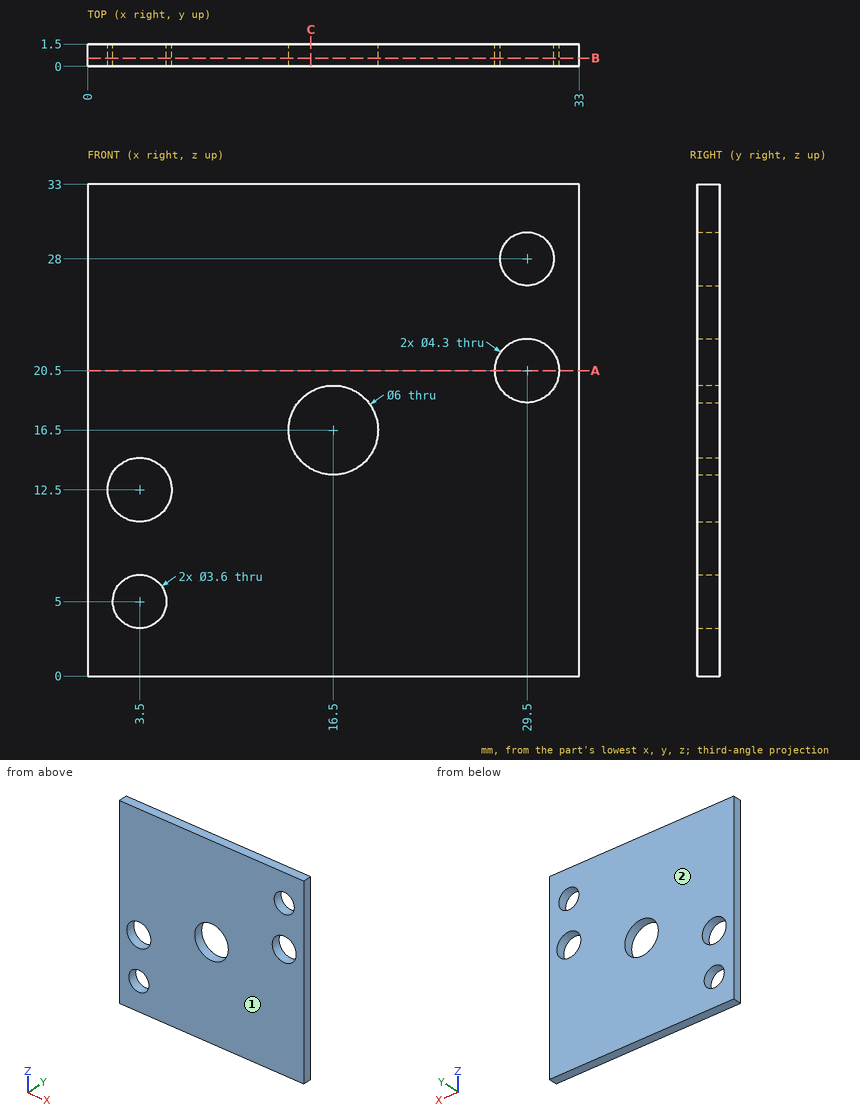
Check sheet for the drawn part. Datum: minimum x, y, z corner. Units: mm. Round coordinates to 2 decimals unless told otherwise and drop trailing zeros. Loops run counter-clockwise (first coordinate to the right, second up) from the corner with the lowest first, then second, coordinate; pieces in that order, holes last.
Item 1: Mould release check, pull along Y, two halves, no side actions. Record for the marked faces 1 and 2: pulls with the +Y half, pulls with the -Y half, needs draft (parallel to the pull), parting line crosses it, or undercut.
Item 2: Gauge pin test, flat ends, axial feed: pin 1 (4 mm diameter, centred on x = 29.5, z = 20.5, fed in from -Y); pin 2 (6 mm diameter, centred on x = 3.5, z = 5, fed in from -Y). Record the tip position at first contact, or that the pin passes through.
Item 3: Cross-section at B-B on y = 0.55. Record the boundary of the cut face in (x, z).
Item 4: Thickness scan on line 1 (Z direction, x = 29.5, y = 0.55); line 2 (X direction, y = 0.9, z = 5); line 3 (X direction, y = 0.9, z = 16.5). Record the ranges inside material, lowest first.
Item 5: Cross-section at A-A on z = 20.5. Record the boundary of the cut face in (x, y).
Item 6: Cross-section at C-C on x = 15. Record the boundary of the cut face in (y, z), then the cut area to 3 significant figures.
Answer sheet:
1. face 1: pulls with the -Y half
1. face 2: pulls with the +Y half
2. pin 1: passes through
2. pin 2: stops at y = 0
3. outline: (0, 0) - (33, 0) - (33, 33) - (0, 33) - close; hole circle Ø4.3 at (3.5, 12.5); hole circle Ø3.6 at (3.5, 5); hole circle Ø6 at (16.5, 16.5); hole circle Ø4.3 at (29.5, 20.5); hole circle Ø3.6 at (29.5, 28)
4. line 1: z = 0 to 18.35, 22.65 to 26.2, 29.8 to 33
4. line 2: x = 0 to 1.7, 5.3 to 33
4. line 3: x = 0 to 13.5, 19.5 to 33
5. outline: (0, 0) - (27.35, 0) - (27.35, 1.5) - (0, 1.5) - close; (31.65, 0) - (33, 0) - (33, 1.5) - (31.65, 1.5) - close
6. outline: (0, 0) - (1.5, 0) - (1.5, 13.9) - (0, 13.9) - close; (0, 19.1) - (1.5, 19.1) - (1.5, 33) - (0, 33) - close
6. area: 41.7 mm2
